Read the model definition and answer for the solid it produces. Units are mm, in the model's axes. A direction names the side the tool comes from. Coordinates: 2 decimals unless noted, no trailing zeros. Order: outer loops, then holes, each group sorted by start corner. A loop starts at its lowest first (then second) coordinate and runs counter-clockwise, first axis right, second up. Notation, with made-up numbers: (-40, 55) -> (-17, 55) arc R21 cw to (-17, 60) -> close; hole circle Ø11 at (46.5, -1). An arc over 180 degrees is marked (long way). Answer in a Markdown table with one row per item.
from build123d import *

# Parameters (mm, degrees)
SKETCH_1_W          = 60
SKETCH_1_H          = 30
EXTRUDE_1_DEPTH     = 10
EXTRUDE_2_DEPTH     = 20
SKETCH_3_W          = 60
SKETCH_3_H          = 30
SKETCH_3_W_2        = 56
SKETCH_3_H_2        = 26
EXTRUDE_3_DEPTH     = 4
SKETCH_4_R          = 1
EXTRUDE_4_DEPTH     = 37
SKETCH_5_W          = 66
SKETCH_5_H          = 36
EXTRUDE_5_DEPTH     = 4
CUT_EXTRUDE_1_REACH = 98.348
SKETCH_6_R          = 5


with BuildPart() as part:
    # 草图1 → 凸台-拉伸1 (new body)
    with BuildSketch(Plane(origin=(0, 0, 0), x_dir=(1, 0, 0), z_dir=(0, 1, 0))):
        with Locations((30, 15)):
            Rectangle(SKETCH_1_W, SKETCH_1_H)
    extrude(amount=EXTRUDE_1_DEPTH)

    # 草图2 → 凸台-拉伸2 (add)
    with BuildSketch(Plane(origin=(0, 10, 0), x_dir=(1, 0, 0), z_dir=(0, 1, 0))):
        Polygon((60, 0), (51, 0), (51, 2), (58, 2), (58, 28), (2, 28), (2, 2), (9, 2), (9, 0), (0, 0), (0, 30), (60, 30), align=None)
    extrude(amount=EXTRUDE_2_DEPTH)

    # 草图3 → 凸台-拉伸3 (add)
    with BuildSketch(Plane(origin=(0, 30, 0), x_dir=(1, 0, 0), z_dir=(0, 1, 0))):
        with Locations((30, 15)):
            Rectangle(SKETCH_3_W, SKETCH_3_H)
        with Locations((30, 15)):
            Rectangle(SKETCH_3_W_2, SKETCH_3_H_2, mode=Mode.SUBTRACT)
    extrude(amount=EXTRUDE_3_DEPTH)

    # 草图4 → 凸台-拉伸4 (add)
    with BuildSketch(Plane(origin=(0, 34, 0), x_dir=(1, 0, 0), z_dir=(0, 1, 0))):
        with Locations(Location((1, 29, 0), (0, 0, 90))):
            Circle(SKETCH_4_R)
        with Locations(Location((1, 1, 0), (0, 0, 270))):
            Circle(SKETCH_4_R)
        with Locations(Location((59, 29, 0), (0, 0, 90))):
            Circle(SKETCH_4_R)
        with Locations(Location((59, 1, 0), (0, 0, 270))):
            Circle(SKETCH_4_R)
    extrude(amount=EXTRUDE_4_DEPTH)

    # 草图5 → 凸台-拉伸5 (add)
    with BuildSketch(Plane(origin=(0, 71, 0), x_dir=(1, 0, 0), z_dir=(0, 1, 0))):
        with Locations((30, 15)):
            Rectangle(SKETCH_5_W, SKETCH_5_H)
    extrude(amount=EXTRUDE_5_DEPTH)

    # 草图6 → 切除-拉伸1 (cut, up to next)
    with BuildSketch(Plane(origin=(0, 10, 0), x_dir=(1, 0, 0), z_dir=(0, 1, 0)), mode=Mode.PRIVATE) as cut_extrude_1_sk1:
        with Locations(Location((52.583011954, 22.907401762, 0), (0, 0, 270))):
            Circle(SKETCH_6_R)
    cut_extrude_1_tool1 = extrude(cut_extrude_1_sk1.sketch, amount=-CUT_EXTRUDE_1_REACH, mode=Mode.PRIVATE) & part.part
    add(cut_extrude_1_tool1.solids().sort_by_distance((52.583012, 10, -22.907402))[0], mode=Mode.SUBTRACT)


solid = part.part
Q1. For faces 5 (the face through (30, 9, 0)), 6 (the face through (30, 30, -1)), 7 (the face through (58.16, 52.24, -29.54)), 8 (the face through (0, 17, -15)), 9 (the face through (30, 17, -30)), determine the directions among +Z, -Z, +X, -X, +Y, -Y from which every point of the face is accessible in a straight line to the end or side of a thin tool.
Outcome:
| item | result |
|---|---|
| face 5 | +Z, +X, -X, -Y |
| face 6 | +Z |
| face 7 | none |
| face 8 | +Z, -Z, -X, -Y |
| face 9 | -Z, +X, -X, -Y |
Q2. For a pull along Y with two mould halves and no side action, classify faces 1 (the face through (60, 17, -15)), 2 (the face through (30, 75, -15)), 3 (the face through (0, 52, -1)), 4 (the face through (58, 22, -15)) as pulls with the +Y half, pulls with the -Y half, needs draft (parallel to the pull), parting line crosses it, or undercut.
Outcome:
| item | result |
|---|---|
| face 1 | needs draft |
| face 2 | pulls with the +Y half |
| face 3 | undercut |
| face 4 | undercut |
Q3. The part is cut by section C-C (x = 23). Write down the section's boundary in (y, z), then the cut area to 3 significant figures.
Outcome:
| item | result |
|---|---|
| outline | (0, -30) -> (34, -30) -> (34, -28) -> (10, -28) -> (10, 0) -> (0, 0) -> close; (30, -2) -> (34, -2) -> (34, 0) -> (30, 0) -> close; (71, -33) -> (75, -33) -> (75, 3) -> (71, 3) -> close |
| area | 500 mm² |
Q4. The part is cut by section D-D (z = -25.5). Write down the section's boundary in (x, y), then the cut area to 3 significant figures.
Outcome:
| item | result |
|---|---|
| outline | (-3, 71) -> (63, 71) -> (63, 75) -> (-3, 75) -> close; (0, 0) -> (48.31, 0) -> (48.31, 10) -> (2, 10) -> (2, 34) -> (0, 34) -> close; (56.86, 0) -> (60, 0) -> (60, 34) -> (58, 34) -> (58, 10) -> (56.86, 10) -> close |
| area | 874 mm² |
Q5. The part is cut by section A-A (x = 3). Write down the section's boundary in (y, z).
Outcome:
| item | result |
|---|---|
| outline | (0, -30) -> (34, -30) -> (34, -28) -> (10, -28) -> (10, -2) -> (34, -2) -> (34, 0) -> (0, 0) -> close; (71, -33) -> (75, -33) -> (75, 3) -> (71, 3) -> close |
Q6. Given pin 1 (2 mm diameter, centred on y = 27.5, z = -4.5, fed in from -X); pin 2 (6 mm diameter, centred on x = 51.5, z = -22.5, fed in from -Y); pin 3 (1.6 mm diameter, centred on y = 15, z = -0.5, fed in from +X), each flat-ended and moving along its own axis, determine where each tip first touches the part or whether it passes through.
Outcome:
| item | result |
|---|---|
| pin 1 | x = 0 |
| pin 2 | y = 71 |
| pin 3 | x = 60 |
Q7. Consider line 1 (Y direction, x = 22.5, z = -11.5); line 2 (X direction, y = 21.5, z = -24); line 3 (Z direction, x = 55, y = 15). Determine where each line is inside the solid, lowest interval first.
Outcome:
| item | result |
|---|---|
| line 1 | 0 to 10, 71 to 75 |
| line 2 | 0 to 2, 58 to 60 |
| line 3 | -30 to -28, -2 to 0 |
Q8. The part is cut by section B-B (z = -14). Write down the section's boundary in (x, y).
Outcome:
| item | result |
|---|---|
| outline | (-3, 71) -> (63, 71) -> (63, 75) -> (-3, 75) -> close; (0, 0) -> (60, 0) -> (60, 34) -> (58, 34) -> (58, 10) -> (2, 10) -> (2, 34) -> (0, 34) -> close |
